Design review of the part shown in the three views and the two pictorial views. Dimensions are in mm from the part's minimum x, y and z. A direction names the side the tool comes from. Give positions to 0.01 mm unless a question says otherwise; leave off trailing zeros. Order: outer loops, then holes, each group sorted by start corner. A loop starts at its lowest first (then second) coordinate and runs counter-clockwise, first axis right, second up. Notation, with made-up numbers: (-29.5, 72.25) - (19.5, 72.25) arc R15 cw to (19.5, 80.25) - close; hole circle Ø10 at (53, -20.5). An arc over 180 degrees is marked (long way). Put each result on its own line as item: value.
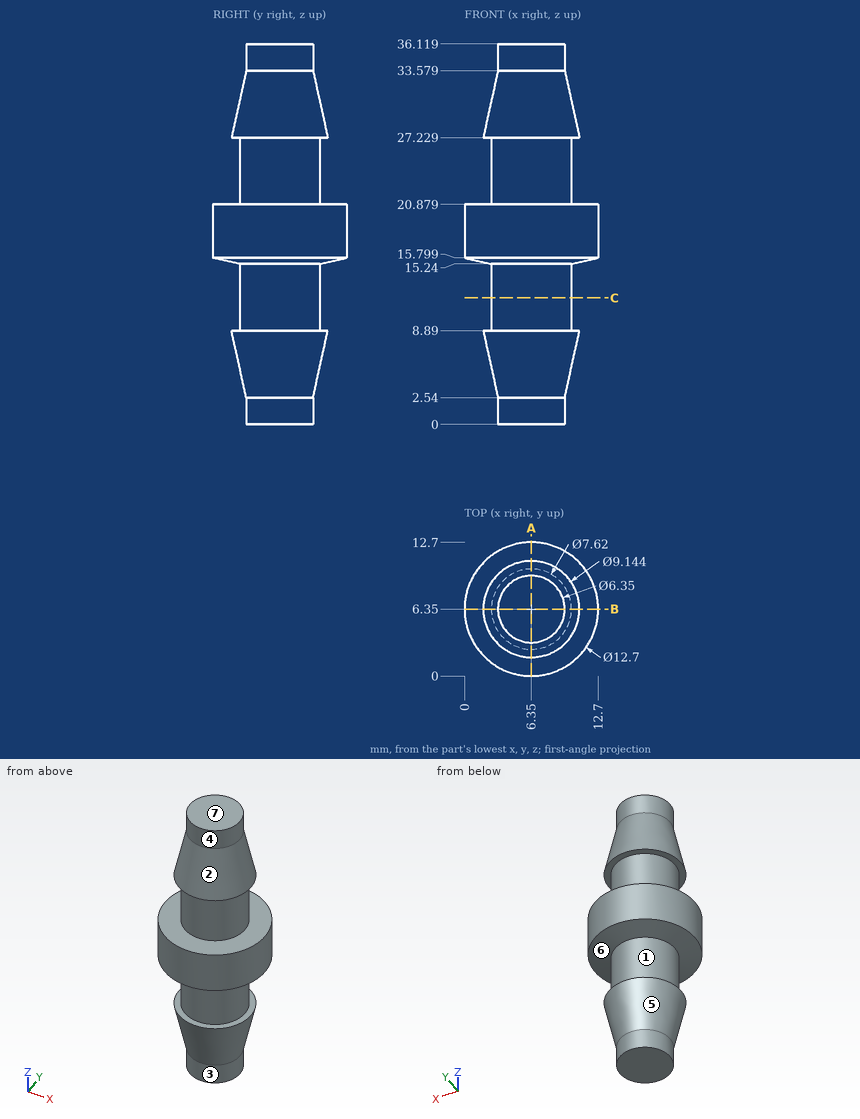
(1) Take a section at A-A, the plane x = 6.35. Write out the cut boundary in (y, z) (1 decimal), then the cut area to 3 significant figures.
The answers:
outline: (0, 15.8) - (2.5, 15.2) - (2.5, 8.9) - (1.8, 8.9) - (3.2, 2.5) - (3.2, 0) - (9.5, 0) - (9.5, 2.5) - (10.9, 8.9) - (10.2, 8.9) - (10.2, 15.2) - (12.7, 15.8) - (12.7, 20.9) - (10.2, 20.9) - (10.2, 27.2) - (10.9, 27.2) - (9.5, 33.6) - (9.5, 36.1) - (3.2, 36.1) - (3.2, 33.6) - (1.8, 27.2) - (2.5, 27.2) - (2.5, 20.9) - (0, 20.9) - close
area: 298 mm^2
(2) Take a section at C-C, the plane z = 12. Write out the cut boundary in (x, y).
The answers:
outline: circle Ø7.62 at (6.35, 6.35)
(3) For the marked faces 1, 2 and 3, list the 3-axis set-ups (+Z, -Z, +X, -X, +Y, -Y) from which the entire face can be reached by the end or side of a thin tool; tool diameter is ignored.
The answers:
face 1: none
face 2: +Z
face 3: -Z
(4) Wall thickness on L1, parallel to X at y = 5, z = 3.5 (1 decimal); L2, parallel to X at y = 7, z = 27; L3, parallel to Y at x = 10, z = 8.5: over which ranges is each line inside the solid? List them lowest first.
The answers:
L1: 3.2 to 9.5
L2: 2.6 to 10.1
L3: 3.74 to 8.96
(5) The part is to be moulded in two halves that separate along Z. For the marked faces 4, 5, 6 and 7, say which applies: pulls with the +Z half, pulls with the -Z half, needs draft (parallel to the pull), parting line crosses it, or undercut.
The answers:
face 4: needs draft
face 5: pulls with the -Z half
face 6: undercut
face 7: pulls with the +Z half
(6) Clearance check with flat-ended pins moving along their axes: pin 1 Ø1.5 at (x, z) = (5.5, 12) entering from +Y; pin 2 Ø3 at (y, z) = (9, 12.5) entering from +X; pin 3 Ø4 at (x, z) = (3.5, 15.5) entering from +Y. State where each tip first meets the part, or that it passes through.
The answers:
pin 1: y = 10.16
pin 2: x = 9.98
pin 3: y = 12.64
